from build123d import *

# Parameters (mm, degrees)
SKETCH_1_W          = 20
SKETCH_1_H          = 100
SKETCH_1_R          = 1
EXTRUDE_1_DEPTH     = 2
SKETCH_3_R          = 10
CUT_EXTRUDE_2_DEPTH = 10
SKETCH_4_R          = 1
CUT_EXTRUDE_3_DEPTH = 10
FILLET_2_R          = 1
SKETCH_5_R          = 1
CUT_EXTRUDE_4_DEPTH = 103
SKETCH_6_R          = 1.5
CUT_EXTRUDE_5_DEPTH = 1


with BuildPart() as part:
    # 草图1 → 凸台-拉伸1 (new body)
    with BuildSketch(Plane(origin=(0, 0, 0), x_dir=(0, 0, -1), z_dir=(1, 0, 0))):
        with Locations((10, 50)):
            Rectangle(SKETCH_1_W, SKETCH_1_H)
        with Locations((2.5, 97.5)):
            Circle(SKETCH_1_R, mode=Mode.SUBTRACT)
        with Locations((17.5, 97.5)):
            Circle(SKETCH_1_R, mode=Mode.SUBTRACT)
        with Locations((17.5, 82.5)):
            Circle(SKETCH_1_R, mode=Mode.SUBTRACT)
        with Locations((2.5, 82.5)):
            Circle(SKETCH_1_R, mode=Mode.SUBTRACT)
        with Locations(Location((17.5, 17.5, 0), (0, 0, 180))):
            Circle(SKETCH_1_R, mode=Mode.SUBTRACT)
        with Locations(Location((2.5, 17.5, 0), (0, 0, 180))):
            Circle(SKETCH_1_R, mode=Mode.SUBTRACT)
        with Locations(Location((2.5, 2.5, 0), (0, 0, 180))):
            Circle(SKETCH_1_R, mode=Mode.SUBTRACT)
        with Locations(Location((17.5, 2.5, 0), (0, 0, 180))):
            Circle(SKETCH_1_R, mode=Mode.SUBTRACT)
    extrude(amount=EXTRUDE_1_DEPTH)

    # 草图3 → 切除-拉伸2 (cut)
    with BuildSketch(Plane(origin=(2, 0, 0), x_dir=(0, 0, -1), z_dir=(1, 0, 0))):
        with Locations((10, 109)):
            Circle(SKETCH_3_R)
        with Locations((-9, 90)):
            Circle(SKETCH_3_R)
        with Locations((29, 90)):
            Circle(SKETCH_3_R)
    cut_extrude_2 = extrude(amount=-CUT_EXTRUDE_2_DEPTH, mode=Mode.SUBTRACT)

    # 镜向2: 切除-拉伸2 across plane
    add(cut_extrude_2.mirror(Plane(origin=(0, 50, 0), x_dir=(0, 0, 1), z_dir=(0, -1, 0))), mode=Mode.SUBTRACT)

    # 草图4 → 切除-拉伸3 (cut)
    with BuildSketch(Plane(origin=(2, 0, 0), x_dir=(0, 0, -1), z_dir=(1, 0, 0))):
        with Locations((10, 97)):
            Circle(SKETCH_4_R)
        with Locations((3, 90)):
            Circle(SKETCH_4_R)
        with Locations((17, 90)):
            Circle(SKETCH_4_R)
        with Locations((10, 83)):
            Circle(SKETCH_4_R)
    cut_extrude_3 = extrude(amount=-CUT_EXTRUDE_3_DEPTH, mode=Mode.SUBTRACT)

    # 镜向3: 切除-拉伸3 across plane
    add(cut_extrude_3.mirror(Plane(origin=(0, 50, 0), x_dir=(0, 0, 1), z_dir=(0, -1, 0))), mode=Mode.SUBTRACT)

    # 圆角2
    fillet_2_edges = [part.edges().sort_by_distance(p)[0] for p in [
        (1, 100, -5.641101056),
        (1, 100, -14.358898944),
        (1, 85.641101056, 0),
        (1, 94.358898944, 0),
        (1, 94.358898944, -20),
        (1, 85.641101056, -20),
        (1, 100, 0),
        (1, 0, -14.358898944),
        (1, 100, -20),
        (1, 0, -5.641101056),
        (1, 0, -20),
        (1, 0, 0),
        (1, 5.641101056, 0),
        (1, 14.358898944, 0),
        (1, 14.358898944, -20),
        (1, 5.641101056, -20),
    ]]
    fillet(fillet_2_edges, radius=FILLET_2_R)

    # 草图5 → 切除-拉伸4 (cut, through all)
    with BuildSketch(Plane.ZY):
        with Locations((-10, 60)):
            Circle(SKETCH_5_R)
        with Locations((-10, 40)):
            Circle(SKETCH_5_R)
    extrude(amount=-CUT_EXTRUDE_4_DEPTH, mode=Mode.SUBTRACT)

    # 草图6 → 切除-拉伸5 (cut)
    with BuildSketch(Plane.ZY):
        with Locations((-2.5, 97.5)):
            Circle(SKETCH_6_R)
        with Locations((-3, 90)):
            Circle(SKETCH_6_R)
        with Locations((-2.5, 82.5)):
            Circle(SKETCH_6_R)
        with Locations((-10, 97)):
            Circle(SKETCH_6_R)
        with Locations((-10, 83)):
            Circle(SKETCH_6_R)
        with Locations((-17.5, 97.5)):
            Circle(SKETCH_6_R)
        with Locations((-17, 90)):
            Circle(SKETCH_6_R)
        with Locations((-17.5, 82.5)):
            Circle(SKETCH_6_R)
        with Locations((-10, 60)):
            Circle(SKETCH_6_R)
        with Locations((-10, 40)):
            Circle(SKETCH_6_R)
        with Locations((-2.5, 17.5)):
            Circle(SKETCH_6_R)
        with Locations((-3, 10)):
            Circle(SKETCH_6_R)
        with Locations((-2.5, 2.5)):
            Circle(SKETCH_6_R)
        with Locations((-10, 17)):
            Circle(SKETCH_6_R)
        with Locations((-10, 3)):
            Circle(SKETCH_6_R)
        with Locations((-17.5, 17.5)):
            Circle(SKETCH_6_R)
        with Locations((-17, 10)):
            Circle(SKETCH_6_R)
        with Locations((-17.5, 2.5)):
            Circle(SKETCH_6_R)
    extrude(amount=-CUT_EXTRUDE_5_DEPTH, mode=Mode.SUBTRACT)


solid = part.part
Can you work these out from the model? Positions are in its coordinate system, mm. A direction names the side the tool comes from. Coordinates: 2 decimals unless noted, no trailing zeros. Write each loop counter-clockwise with the first axis right and the second up, starting at its lowest first coordinate (ties: lowest second). Pieces come first, ordered by that corner, then holes. Notation, with made-up numbers: (73, -37) -> (121, -37) arc R19 ccw to (121, -8) -> close; hole circle Ø3 at (14, 1.5). An arc over 180 degrees is marked (long way). Write item = value, one per line.
(1) Thinking about a two-plate mould opening in Z: for faces 1 (the face through (1, 97, -20)), 2 (the face through (1.51, 96.11, -10.46)), 3 (the face through (1, 90, -1)), 4 (the face through (0.493, 38.536, -10.325)), which applies, +Z half, -Z half, draft (parallel to the pull), parting line (faces both ways), or undercut?
Verdict:
face_1 = -Z half
face_2 = undercut
face_3 = +Z half
face_4 = undercut
(2) Imagine slicing it at B-B (x = 1.7). State how many separate pieces and enclosed holes the cut face has, and give its area (3 significant figures).
Verdict:
separate_pieces = 1
enclosed_holes = 18
area = 1,910 mm^2
(3) For pin 1 (1.5 mm diameter, centred on y = 18, z = -2, fed in from -X), with a flat end and sliding along its axis, tell me the tip position at first contact or that it passes through.
Verdict:
pin_1 = 1
(4) On a 3-axis mill with a long thin cutter (end or side, diameter ignored), from which of +Z, -Z, +X, -X, +Y, -Y can I reach the whole of each face in a straight line? I mean faces 5 (the face through (0.493, 83.987, -17.695)), 6 (the face through (1.49, 81.61, -17.96)). Say none if no direction works.
Verdict:
face_5 = -X
face_6 = +X, -X
(5) Imagine slicing it at A-A (y = 40). Please give me the cut outline in (x, z).
Verdict:
outline = (0, -20) -> (2, -20) -> (2, -11) -> (1, -11) -> (1, -11.5) -> (0, -11.5) -> close; (0, -8.5) -> (1, -8.5) -> (1, -9) -> (2, -9) -> (2, 0) -> (0, 0) -> close
(6) If I drill on probe 1 along Z at (x, y) = (1.7, 90); probe 2 along Z at (x, y) = (0.5, 90); probe 3 along Z at (x, y) = (0.8, 82.5), over which ranges is the centre line in solid material (lowest first)?
Verdict:
probe_1 = -19 to -18, -16 to -4, -2 to -1
probe_2 = -19 to -18.5, -15.5 to -4.5, -1.5 to -1
probe_3 = -20 to -19, -16 to -11.41, -8.59 to -4, -1 to 0
